Geometry: final body of the model. Coordinates: model frame, mm. A direction names the side the tool comes from. Round coordinates to 2 decimals unless told otherwise and drop trailing zeros. Order: outer loops, then holes, each group sorted by start corner. A loop starts at its lowest first (then second) coordinate and runs counter-clockwise, first axis right, second up. Notation, with made-up numbers: (-11.5, -16) -> (42.5, -16) arc R16 ccw to (42.5, 9) -> close; hole circle Ø9 at (1.25, 10). An arc over 180 degrees is marked (long way). Put each result on its own line as item: value.
```python
from build123d import *

# Parameters (mm, degrees)
SKETCH1_R           = 14
SKETCH1_R_2         = 13
BOSS_EXTRUDE1_DEPTH = 1
SKETCH2_R           = 4
BOSS_EXTRUDE2_DEPTH = 4
BOSS_EXTRUDE3_START = 16
SKETCH2_4_R         = 14
SKETCH2_4_R_2       = 13
BOSS_EXTRUDE3_DEPTH = 16
FILLET1_R           = 4
FILLET2_R           = 0.5
FILLET3_R           = 1


with BuildPart() as part:
    # Sketch1 → Boss-Extrude1 (new body)
    # profile 1 of 2: a face of its own
    with BuildSketch(Plane(origin=(0, 0, 0), x_dir=(1, 0, 0), z_dir=(0, 1, 0))):
        with Locations(Location((0, 0, 0), (0, 0, 270))):
            Circle(SKETCH1_R)
        Circle(SKETCH1_R_2, mode=Mode.SUBTRACT)
    # profile 2 of 2: a face of its own
    with BuildSketch(Plane(origin=(0, 0, 0), x_dir=(1, 0, 0), z_dir=(0, 1, 0))):
        Circle(SKETCH1_R_2)
    extrude(amount=BOSS_EXTRUDE1_DEPTH)

    # Sketch2 → Boss-Extrude2 (add)
    with BuildSketch(Plane.XZ):
        with Locations(Location((0, 0, 0), (0, 0, 270))):
            Circle(SKETCH2_R)
    extrude(amount=BOSS_EXTRUDE2_DEPTH)

    # Sketch2<4> → Boss-Extrude3 (add)
    with BuildSketch(Plane.XZ.offset(BOSS_EXTRUDE3_START)):
        with Locations(Location((0, 0, 0), (0, 0, 270))):
            Circle(SKETCH2_4_R)
        with Locations(Location((0, 0, 0), (0, 0, 270))):
            Circle(SKETCH2_4_R_2, mode=Mode.SUBTRACT)
    extrude(amount=-BOSS_EXTRUDE3_DEPTH)

    # Fillet1
    fillet1_edges = [part.edges().sort_by_distance(p)[0] for p in [
        (0, 0, 4),
    ]]
    fillet(fillet1_edges, radius=FILLET1_R - 0.0001)  # a hair under: the kernel refuses the full size

    # Fillet2
    fillet2_edges = [part.edges().sort_by_distance(p)[0] for p in [
        (0, -4, 4),
    ]]
    fillet(fillet2_edges, radius=FILLET2_R)

    # Fillet3
    fillet3_edges = [part.edges().sort_by_distance(p)[0] for p in [
        (0, 0, 13),
        (0, 1, -14),
    ]]
    fillet(fillet3_edges, radius=FILLET3_R - 0.0001)  # a hair under: the kernel refuses the full size


solid = part.part
```
1. Cut plane A-A on y = -5. Return loops of the section in (x, z), and give its area (3 significant figures).
Ans:
outline: circle Ø28 at (0, 0); hole circle Ø26 at (0, 0)
area: 84.8 mm²
2. Draft query along Z for faces 3 (the face through (2, 0, 8)), 4 (the face through (0, 1, 0)), 5 (the face through (-7.91, -8.605, 10.316)). Return one class per face: +Z half, -Z half, draft (parallel to the pull), parting line (faces both ways), or undercut.
Ans:
face 3: undercut
face 4: draft
face 5: undercut
3. Material intervals for probe 1 along X at (y, z) = (-8.25, 0); probe 2 along Y at (x, z) = (9.75, -5.5); probe 3 along Z at (x, y) = (3.25, -9.25), sorted ascending.
Ans:
probe 1: -14 to -13, 13 to 14
probe 2: 0 to 1
probe 3: -13.62 to -12.59, 12.59 to 13.62
4. Set-up query: faces 1 (the face through (-9.3, -16, -9.3)), 2 (the face through (0, -4, 0)). Return all of +Z, -Z, +X, -X, +Y, -Y with unobstructed straight access to the full face (end or side cutting, diameter ignored); none if empty.
Ans:
face 1: +Z, -Z, +X, -X, -Y
face 2: -Y
5. Contact query for flat-ended pins moving along their axis: P1, Ø8, axis at x = -0.5, z = 1, coming from the -Y side; P2, Ø1.5, axis at y = -11, z = -5.5, coming from the -X side; P3, Ø4, axis at x = -3.5, y = -9.5, coming from the -Z side. Output: stop coordinate, or through.
Ans:
P1: y = -4
P2: x = -13.17
P3: z = -13.92
6. Cut plane B-B on y = -2.75. Return loops of the section in (x, z), and give its area (3 significant figures).
Ans:
outline: circle Ø28 at (0, 0); circle Ø8.4 at (0, 0); hole circle Ø26 at (0, 0)
area: 140 mm²
